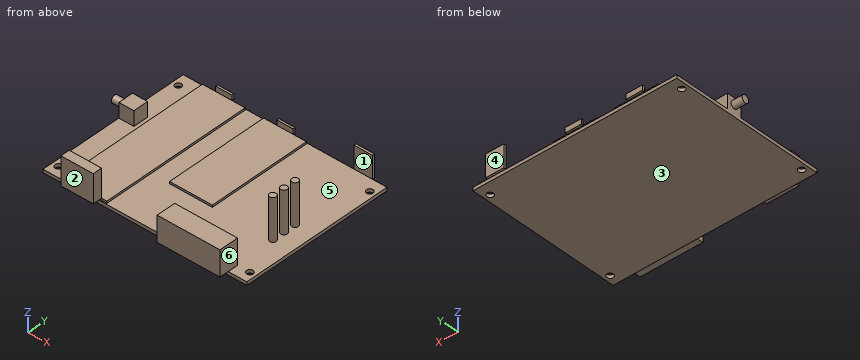
```python
from build123d import *

# Parameters (mm, degrees)
SKETCH_W     = 100
SKETCH_H     = 76
SKETCH_R     = 1.6
PAD_DEPTH    = 1.6
SKETCH001_W  = 21
SKETCH001_H  = 75
PAD001_DEPTH = 1
SKETCH002_W  = 15.9
SKETCH002_H  = 4.5
PAD002_DEPTH = 13.85
SKETCH003_W  = 8
SKETCH003_H  = 1
PAD003_DEPTH = 2.5
SKETCH004_W  = 30.84
SKETCH004_H  = 9.52
PAD004_DEPTH = 12.5
SKETCH005_W  = 21
SKETCH005_H  = 51
PAD005_DEPTH = 1
SKETCH006_W  = 8
SKETCH006_H  = 1
PAD006_DEPTH = 2.5
SKETCH007_W  = 9
SKETCH007_H  = 1.1
PAD007_DEPTH = 11
SKETCH008_W  = 7.4
SKETCH008_H  = 7.4
PAD008_DEPTH = 7.2
SKETCH009_R  = 1.8
PAD009_DEPTH = 5.4
SKETCH010_R  = 1.6
PAD010_DEPTH = 20.5


with BuildPart() as part:
    # Sketch → Pad (new body)
    with BuildSketch(Plane.XY):
        Rectangle(SKETCH_W, SKETCH_H)
        with Locations((-47, 32)):
            Circle(SKETCH_R, mode=Mode.SUBTRACT)
        with Locations((47, 32)):
            Circle(SKETCH_R, mode=Mode.SUBTRACT)
        with Locations((-47, -33)):
            Circle(SKETCH_R, mode=Mode.SUBTRACT)
        with Locations((47, -33)):
            Circle(SKETCH_R, mode=Mode.SUBTRACT)
    extrude(amount=PAD_DEPTH)

    # Sketch001 → Pad001 (join)
    with BuildSketch(Plane.XY.offset(1.6)):
        with Locations((-29.65, 0.02)):
            Rectangle(SKETCH001_W, SKETCH001_H)
    extrude(amount=PAD001_DEPTH)

    # Sketch002 → Pad002 (join)
    with BuildSketch(Plane.XY.offset(2.59)):
        with Locations((-29.65, -39.73)):
            Rectangle(SKETCH002_W, SKETCH002_H)
    extrude(amount=PAD002_DEPTH)

    # Sketch003 → Pad003 (join)
    with BuildSketch(Plane.XY.offset(2.599)):
        with Locations((-29.65, 38.02)):
            Rectangle(SKETCH003_W, SKETCH003_H)
    extrude(amount=PAD003_DEPTH)

    # Sketch004 → Pad004 (join)
    with BuildSketch(Plane.XY.offset(1.6)):
        with Locations((25.46, -37.69)):
            Rectangle(SKETCH004_W, SKETCH004_H)
    extrude(amount=PAD004_DEPTH)

    # Sketch005 → Pad005 (join)
    with BuildSketch(Plane.XY.offset(1.6)):
        with Locations((0.4, 12.02)):
            Rectangle(SKETCH005_W, SKETCH005_H)
    extrude(amount=PAD005_DEPTH)

    # Sketch006 → Pad006 (join)
    with BuildSketch(Plane.XY.offset(2.599)):
        with Locations((0.4, 38.02)):
            Rectangle(SKETCH006_W, SKETCH006_H)
    extrude(amount=PAD006_DEPTH)

    # Sketch007 → Pad007 (join)
    with BuildSketch(Plane.XY.offset(1.599)):
        with Locations((38.35, 38.55)):
            Rectangle(SKETCH007_W, SKETCH007_H)
    extrude(amount=PAD007_DEPTH)

    # Sketch008 → Pad008 (join)
    with BuildSketch(Plane.XY.offset(1.6)):
        with Locations((-46.3, 6.8)):
            Rectangle(SKETCH008_W, SKETCH008_H)
    extrude(amount=PAD008_DEPTH)

    # Sketch009 → Pad009 (join)
    with BuildSketch(Plane.YZ.offset(-50)):
        with Locations((6.8, 5.5)):
            Circle(SKETCH009_R)
    extrude(amount=-PAD009_DEPTH)

    # Sketch010 → Pad010 (join)
    with BuildSketch(Plane.XY.offset(1.6)):
        with Locations((40.2, -1)):
            Circle(SKETCH010_R)
        with Locations((40.2, -7)):
            Circle(SKETCH010_R)
        with Locations((40.2, -13)):
            Circle(SKETCH010_R)
    extrude(amount=PAD010_DEPTH)


solid = part.part
```
Geometry check sheet. Reference: the model listing, model coordinates, mm. Face numbers are marked on the shaded views. A direction names the side the tool comes from. Coordinates: 2 decimals unless noted, no trailing zeros. Order: outer loops, then holes, each group sorted by start corner. A loop starts at its lowest first (then second) coordinate and runs counter-clockwise, first axis right, second up.
Q1. Sectioned sample at C-C on y = -24.5. Record the cut outline in (x, z).
Reply:
outline: (-50, 0) - (50, 0) - (50, 1.6) - (-19.15, 1.6) - (-19.15, 2.6) - (-40.15, 2.6) - (-40.15, 1.6) - (-50, 1.6) - close
Q2. Depth check by flat-ended pin: pin 1 Ø2 at (y, z) = (-40.5, 12) entering from -X; pin 2 Ø5 at (x, y) = (-26.5, -6.5) entering from +Z; pin 3 Ø12 at (x, z) = (26.5, 14) entering from +Y. Enter the tip coordinate at first touch or a pass-through.
Reply:
pin 1: stops at x = -37.6
pin 2: stops at z = 2.6
pin 3: stops at y = -32.93
Q3. Sectioned sample at B-B on x = 35. Record the cut outline in (y, z), and give its area (3 significant figures).
Reply:
outline: (-42.45, 1.6) - (-38, 1.6) - (-38, 0) - (38, 0) - (38, 1.6) - (39.1, 1.6) - (39.1, 12.6) - (38, 12.6) - (38, 1.6) - (-32.93, 1.6) - (-32.93, 14.1) - (-42.45, 14.1) - close
area: 253 mm2
Q4. Sectioned sample at A-A on z = 10.75. Record the cut outline in (x, y), and give its area (3 significant figures).
Reply:
outline: (-37.6, -41.98) - (-21.7, -41.98) - (-21.7, -37.48) - (-37.6, -37.48) - close; (10.04, -42.45) - (40.88, -42.45) - (40.88, -32.93) - (10.04, -32.93) - close; (33.85, 38) - (42.85, 38) - (42.85, 39.1) - (33.85, 39.1) - close; circle Ø3.2 at (40.2, -13); circle Ø3.2 at (40.2, -7); circle Ø3.2 at (40.2, -1)
area: 399 mm2
Q5. Draft check along X on the marked faces 4, 5 and 6. Enter one of: released by +X, released by -X, zero draft, split by the parting line, or undercut.
Reply:
face 4: zero draft
face 5: undercut
face 6: released by +X
Q6. Tool access check on the marked faces 1, 2 and 3. Record the directions out of +Z, -Z, +X, -X, +Y, -Y that give a thin tool (end or side, any length) a straight path to the whole face; none if there is none.
Reply:
face 1: +Z, +X
face 2: +Z, -Z, -X, -Y
face 3: -Z, +X, -X, +Y, -Y
Q7. Thickness scan on probe 1 along Y at (x, z) = (47, 1.15); probe 2 along X at (y, z) = (13.5, 2.5); probe 3 along X at (y, z) = (8, 1.5). Record the ranges inside material, lowest first.
Reply:
probe 1: y = -38 to -34.6, -31.4 to 30.4, 33.6 to 38
probe 2: x = -40.15 to -19.15, -10.1 to 10.9
probe 3: x = -50 to 50
Q8. Sectioned sample at D-D on x = -1.5. Record the cut outline in (y, z), and give its area (3 significant figures).
Reply:
outline: (-38, 0) - (38, 0) - (38, 1.6) - (37.52, 1.6) - (37.52, 2.6) - (38.52, 2.6) - (38.52, 5.1) - (37.52, 5.1) - (37.52, 2.6) - (-13.48, 2.6) - (-13.48, 1.6) - (-38, 1.6) - close
area: 175 mm2
